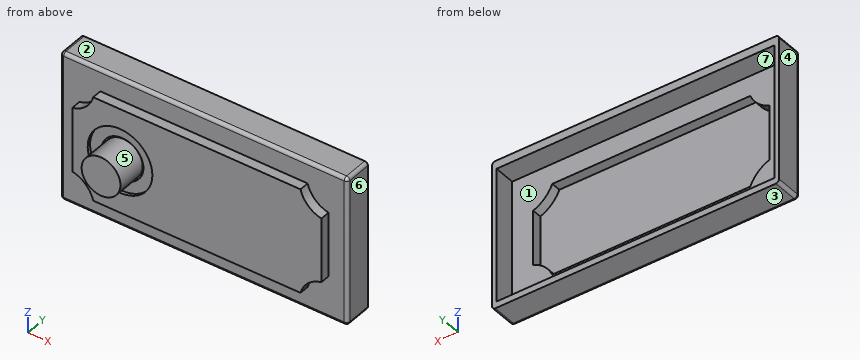
```python
from build123d import *

# Parameters (mm, degrees)
TOP_COVER_SKETCH_01_W       = 44.37
TOP_COVER_SKETCH_01_H       = 23.06
TOP_COVER_EXT_SHAPE_DEPTH   = 4.3
SALIENTE_EXTRUIR1_DEPTH     = 1.5
VACIADO1_T                  = -1
VACIADO1_THICKNESS_2_FACE_W = 21.06
VACIADO1_THICKNESS_2_FACE_H = 3.3
VACIADO1_THICKNESS_2_DEPTH  = 0.31
VACIADO1_THICKNESS_3_FACE_W = 21.06
VACIADO1_THICKNESS_3_FACE_H = 3.3
VACIADO1_THICKNESS_3_DEPTH  = 0.31
VACIADO1_THICKNESS_4_FACE_W = 42.99
VACIADO1_THICKNESS_4_FACE_H = 3.3
VACIADO1_THICKNESS_4_DEPTH  = 0.02
VACIADO1_THICKNESS_5_FACE_W = 42.99
VACIADO1_THICKNESS_5_FACE_H = 3.3
VACIADO1_THICKNESS_5_DEPTH  = 0.3
CROQUIS1_R                  = 3.25
CORTAR_EXTRUIR1_DEPTH       = 0.7
CROQUIS1_5_R                = 5
CROQUIS1_5_R_2              = 3.25
CORTAR_EXTRUIR2_DEPTH       = 0.5
CROQUIS2_R                  = 3
SALIENTE_EXTRUIR2_DEPTH     = 4.7
REDONDEO1_R                 = 0.5


with BuildPart() as part:
    # Top-cover-sketch-01 → Top-cover-ext-shape (new body)
    with BuildSketch(Plane(origin=(0, 0, 0), x_dir=(1, 0, 0), z_dir=(0, 1, 0))):
        Rectangle(TOP_COVER_SKETCH_01_W, TOP_COVER_SKETCH_01_H)
    extrude(amount=TOP_COVER_EXT_SHAPE_DEPTH)

    # Top-cover-sketch-01_18 → Saliente-Extruir1 (add)
    with BuildSketch(Plane(origin=(0, 0, 0), x_dir=(1, 0, 0), z_dir=(0, 1, 0))):
        with BuildLine():
            Line((-19.255, -4.986911136), (-19.255, 4.986911136))
            ThreePointArc((-19.255, 4.986911136), (-17.190017633, 6.076280801), (-16.025784389, 8.1))
            Line((-16.025784389, 8.1), (16.025784389, 8.1))
            ThreePointArc((16.025784389, 8.1), (17.190017633, 6.076280801), (19.255, 4.986911136))
            Line((19.255, 4.986911136), (19.255, -4.986911136))
            ThreePointArc((19.255, -4.986911136), (17.190017633, -6.076280801), (16.025784389, -8.1))
            Line((16.025784389, -8.1), (-16.025784389, -8.1))
            ThreePointArc((-16.025784389, -8.1), (-17.190017633, -6.076280801), (-19.255, -4.986911136))
        make_face()
    extrude(amount=-SALIENTE_EXTRUIR1_DEPTH)

    # Vaciado1
    vaciado1_openings = [part.faces().sort_by_distance(p)[0] for p in [
        (0, 4.3, 0),
    ]]
    offset(amount=VACIADO1_T, openings=vaciado1_openings, kind=Kind.INTERSECTION)

    # Vaciado1 thickness 2 face (on inner face of the shell) → Vaciado1 thickness 2 (cut)
    with BuildSketch(Plane(origin=(-21.185, 2.65, 0), x_dir=(0, 0, -1), z_dir=(-1, 0, 0))):
        Rectangle(VACIADO1_THICKNESS_2_FACE_W, VACIADO1_THICKNESS_2_FACE_H)
    extrude(amount=VACIADO1_THICKNESS_2_DEPTH, mode=Mode.SUBTRACT)

    # Vaciado1 thickness 3 face (on inner face of the shell) → Vaciado1 thickness 3 (cut)
    with BuildSketch(Plane(origin=(21.185, 2.65, 0), x_dir=(0, 0, 1), z_dir=(1, 0, 0))):
        Rectangle(VACIADO1_THICKNESS_3_FACE_W, VACIADO1_THICKNESS_3_FACE_H)
    extrude(amount=VACIADO1_THICKNESS_3_DEPTH, mode=Mode.SUBTRACT)

    # Vaciado1 thickness 4 face (on inner face of the shell) → Vaciado1 thickness 4 (cut)
    with BuildSketch(Plane(origin=(0, 2.65, -10.53), x_dir=(-1, 0, 0), z_dir=(0, 0, -1))):
        Rectangle(VACIADO1_THICKNESS_4_FACE_W, VACIADO1_THICKNESS_4_FACE_H)
    extrude(amount=VACIADO1_THICKNESS_4_DEPTH, mode=Mode.SUBTRACT)

    # Vaciado1 thickness 5 face (on inner face of the shell) → Vaciado1 thickness 5 (add)
    with BuildSketch(Plane(origin=(0, 2.65, 10.53), x_dir=(1, 0, 0), z_dir=(0, 0, 1))):
        Rectangle(VACIADO1_THICKNESS_5_FACE_W, VACIADO1_THICKNESS_5_FACE_H)
    extrude(amount=-VACIADO1_THICKNESS_5_DEPTH)

    # Croquis1 → Cortar-Extruir1 (cut)
    with BuildSketch(Plane.XZ.offset(1.5)):
        with Locations(Location((-11.878900962, 0, 0), (0, 0, 270))):
            Circle(CROQUIS1_R)
    extrude(amount=-CORTAR_EXTRUIR1_DEPTH, mode=Mode.SUBTRACT)

    # Croquis1_5 → Cortar-Extruir2 (cut)
    with BuildSketch(Plane.XZ.offset(1.5)):
        with Locations(Location((-11.878900962, 0, 0), (0, 0, 270))):
            Circle(CROQUIS1_5_R)
        with Locations(Location((-11.878900962, 0, 0), (0, 0, 270))):
            Circle(CROQUIS1_5_R_2, mode=Mode.SUBTRACT)
    extrude(amount=-CORTAR_EXTRUIR2_DEPTH, mode=Mode.SUBTRACT)

    # Croquis2 → Saliente-Extruir2 (add)
    with BuildSketch(Plane.XZ.offset(0.8)):
        with Locations(Location((-11.878900962, 0, 0), (0, 0, 270))):
            Circle(CROQUIS2_R)
    extrude(amount=SALIENTE_EXTRUIR2_DEPTH)

    # Redondeo1
    redondeo1_edges = [part.edges().sort_by_distance(p)[0] for p in [
        (0, 0, -11.53),
        (22.185, 0, 0),
        (0, 0, 11.53),
        (-22.185, 0, 0),
        (-22.185, 2.15, -11.53),
        (22.185, 2.15, -11.53),
        (22.185, 2.15, 11.53),
        (-22.185, 2.15, 11.53),
    ]]
    fillet(redondeo1_edges, radius=REDONDEO1_R)


solid = part.part
```
Geometry: final body of the model. Coordinates: model frame, mm. Face numbers are marked on the shaded views. A direction names the side the tool comes from. Coordinates: 2 decimals unless noted, no trailing zeros. Write each loop counter-clockwise with the first axis right and the second up, starting at its lowest first coordinate (ties: lowest second). Pieces come first, ordered by that corner, then holes. Notation, with made-up numbers: M 51,62 L 88,62 A24 cw 88,73 Z; hole C -24.5,89 d4. An arc over 180 degrees is marked long. Answer as CSV lines item,"result". Start each with the question number.
Q1. Cut plane A-A on y = 1.5. Return the cut outline in (x, z) (3 decimals).
Q2. Line query: line 1 (X direction, y = -0.9, z = 0) (3 decimals); line 2 (X direction, y = -1.4, z = 0) (3 decimals); line 3 (Z direction, x = 3.5, y = 2.25). Output: solid intervals per line, ascending. Write a range as from..to.
Q3. Pin query (flat end, axial travel): P1, Ø13, axis at x = 2.5, z = -1, coming from the -Y side; P2, Ø1.5, axis at x = -7.5, y = -1.5, coming from the -Z side; P3, Ø4.5, axis at x = -6, z = 2.5, coming from the +Y side. Return the tip coordinate at first contact, or that it passes through.
Q4. Cut plane B-B on z = 9.75. Return the cut outline in (x, y) (3 decimals).
Q5. Reachability of the marked faces 5, 6 and 7 from +Z, -Z, +X, -X, +Y, -Y: full face, straight path, thin tool, end or side. Return the list, or none.
Q6. Cut plane C-C on x = 3. Return the cut outline in (y, z), then the cut area to 3 significant figures.
Q7. Mould query, pull axis Z, two halves, no side actions, for the marked faces 1, 2, 3 and 4. Classes: released by +Z, released by -Z, zero draft, split by the parting line, or undercut.
Findings below:
1,outline,"M -22.185,-11.03 A0.5 ccw -21.685,-11.53 L 21.685,-11.53 A0.5 ccw 22.185,-11.03 L 22.185,11.03 A0.5 ccw 21.685,11.53 L -21.685,11.53 A0.5 ccw -22.185,11.03 Z; hole M -21.495,-10.55 L 21.495,-10.55 L 21.495,10.23 L -21.495,10.23 Z"
2,line 1,"x = -19.255..-15.129, -14.879..-8.879, -8.629..19.255"
2,line 2,"x = -19.255..-16.879, -14.879..-8.879, -6.879..19.255"
2,line 3,"z = -11.53..-10.55, 10.23..11.53"
3,P1,"stops at y = -1.5"
3,P2,"stops at z = -8.1"
3,P3,"stops at y = -0.5"
4,outline,"M -22.185,0.5 A0.5 ccw -21.685,0 L 21.685,0 A0.5 ccw 22.185,0.5 L 22.185,4.3 L 21.495,4.3 L 21.495,1 L -21.495,1 L -21.495,4.3 L -22.185,4.3 Z"
5,face 5,"-Y"
5,face 6,"+Z, -Z, +X, +Y, -Y"
5,face 7,"+Y"
6,outline,"M -1.5,-8.1 L 0,-8.1 L 0,-11.03 A0.5 ccw 0.5,-11.53 L 4.3,-11.53 L 4.3,-10.55 L 1,-10.55 L 1,-7.1 L -0.5,-7.1 L -0.5,7.1 L 1,7.1 L 1,10.23 L 4.3,10.23 L 4.3,11.53 L 0.5,11.53 A0.5 ccw 0,11.03 L 0,8.1 L -1.5,8.1 Z"
6,area,"33.5 mm2"
7,face 1,"undercut"
7,face 2,"released by +Z"
7,face 3,"released by -Z"
7,face 4,"zero draft"
